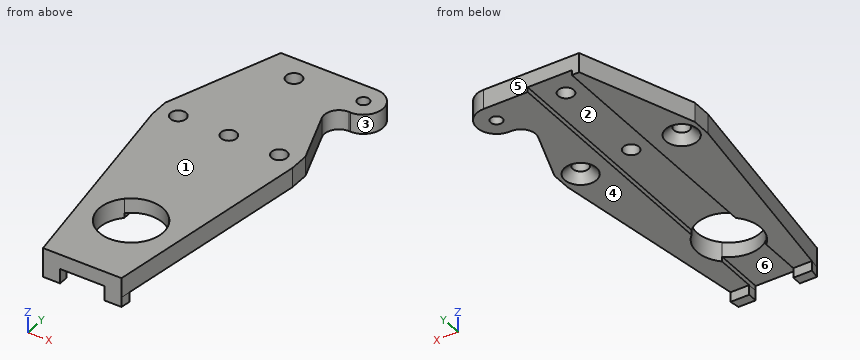
from build123d import *

# Parameters (mm, degrees)
MODEL_R           = 1.2
MODEL_R_2         = 1.6
EXTRUDE_4_DEPTH   = 4
EXTRUDE_4_2_DEPTH = 4
MODEL_7_R         = 1.6
EXTRUDE_5_DEPTH   = 3
EXTRUDE_6_DEPTH   = 6
CHAMFER_2_SIZE    = 1.65


with BuildPart() as part:
    # Model → Extrude 4 (new body)
    with BuildSketch(Plane.XY):
        with BuildLine():
            Line((36.699535099, 24.454545455), (37.040606061, 24.454545455))
            ThreePointArc((37.040606061, 24.454545455), (41.040606061, 28.454545455), (37.040606061, 32.454545455))
            Line((37.040606061, 32.454545455), (28.040606061, 32.454545455))
            Line((28.040606061, 32.454545455), (28.040606061, -17.855038786))
            ThreePointArc((28.040606061, -17.855038786), (30.040606061, -22.545454545), (28.040606061, -27.235870305))
            Line((28.040606061, -27.235870305), (28.040606061, -37.545454545))
            Line((28.040606061, -37.545454545), (31.540606061, -37.545454545))
            Line((31.540606061, -37.545454545), (37.840606061, 5.454545455))
            Line((37.840606061, 5.454545455), (37.840606061, 9.454545455))
            Line((37.840606061, 9.454545455), (33.877655721, 20.43621507))
            ThreePointArc((33.877655721, 20.43621507), (34.244439261, 23.178640702), (36.699535099, 24.454545455))
        make_face()
        with Locations((37.040606061, 28.454545455)):
            Circle(MODEL_R, mode=Mode.SUBTRACT)
        with Locations((33.840606061, 7.454545455)):
            Circle(MODEL_R_2, mode=Mode.SUBTRACT)
    extrude(amount=-EXTRUDE_4_DEPTH)



with BuildPart() as body_2:
    # Model → Extrude 4 2 (new body)
    with BuildSketch(Plane.XY):
        with BuildLine():
            Line((19.040606061, -17.855038786), (19.040606061, 32.454545455))
            Line((19.040606061, 32.454545455), (17.540606061, 32.454545455))
            Line((17.540606061, 32.454545455), (9.240606061, 9.454545455))
            Line((9.240606061, 9.454545455), (9.240606061, 5.454545455))
            Line((9.240606061, 5.454545455), (15.540606061, -37.545454545))
            Line((15.540606061, -37.545454545), (19.040606061, -37.545454545))
            Line((19.040606061, -37.545454545), (19.040606061, -27.235870305))
            ThreePointArc((19.040606061, -27.235870305), (17.040606061, -22.545454545), (19.040606061, -17.855038786))
        make_face()
        with Locations((13.240606061, 7.454545455)):
            Circle(MODEL_R_2, mode=Mode.SUBTRACT)
    extrude(amount=-EXTRUDE_4_2_DEPTH)


with BuildPart() as part_1:
    add(part.part)

    add(body_2.part)  # Extrude 5 merges body 2
    # Model_7 → Extrude 5 (add)
    # profile 1 of 2: a face of its own
    with BuildSketch(Plane.XY):
        with BuildLine():
            Line((28.040606061, -35.545454545), (28.040606061, -27.235870305))
            ThreePointArc((28.040606061, -27.235870305), (23.540606061, -29.045454545), (19.040606061, -27.235870305))
            Line((19.040606061, -27.235870305), (19.040606061, -35.545454545))
            Line((19.040606061, -35.545454545), (19.040606061, -37.545454545))
            Line((19.040606061, -37.545454545), (28.040606061, -37.545454545))
            Line((28.040606061, -37.545454545), (28.040606061, -35.545454545))
        make_face()
    # profile 2 of 2: a face of its own
    with BuildSketch(Plane.XY):
        with BuildLine():
            Line((28.040606061, -17.855038786), (28.040606061, 32.454545455))
            Line((28.040606061, 32.454545455), (19.040606061, 32.454545455))
            Line((19.040606061, 32.454545455), (19.040606061, -17.855038786))
            ThreePointArc((19.040606061, -17.855038786), (23.540606061, -16.045454545), (28.040606061, -17.855038786))
        make_face()
        with Locations((23.540606061, 7.454545455)):
            Circle(MODEL_7_R, mode=Mode.SUBTRACT)
        with Locations((23.540606061, 27.454545455)):
            Circle(MODEL_7_R, mode=Mode.SUBTRACT)
    extrude(amount=-EXTRUDE_5_DEPTH)

    # Model_8 → Extrude 6 (add)
    with BuildSketch(Plane.XY):
        Polygon((31.540606061, -37.545454545), (31.833629316, -35.545454545), (28.04060606, -35.545454545), (28.040606061, -37.545454545), align=None)
        Polygon((19.040606061, -37.545454545), (19.040606061, -35.545454545), (15.247582805, -35.545454545), (15.540606061, -37.545454545), align=None)
    extrude(amount=-EXTRUDE_6_DEPTH)

    # Chamfer 2
    chamfer_2_edges = [part_1.edges().sort_by_distance(p)[0] for p in [
        (32.240606061, 7.454545455, -4),
        (11.640606061, 7.454545455, -4),
    ]]
    chamfer(chamfer_2_edges, length=CHAMFER_2_SIZE)


solid = part_1.part
CAD build for the part. Positions are in the model's coordinates, mm. Face numbers are marked on the shaded views. A direction names the side the tool comes from. Round coordinates to 2 decimals unless told otherwise and drop trailing zeros. Loops run counter-clockwise (first coordinate to the right, second up) from the corner with the lowest first, then second, coordinate; pieces in that order, holes last. Notation, with made-up numbers: (-39, -15.5) - (17, -15.5) arc R7 cw to (17, -10.5) - close; hole circle Ø1 at (-20, -9.5). An arc over 180 degrees is marked (long way). Put each result on its own line as item: value.
1. 3-axis set-ups, long thin cutter, end or side, ignore diameter. For the marked faces 4, 5 and 6: which of +Z, -Z, +X, -X, +Y, -Y reach the whole face in a straight line?
Geometry check:
face 4: -Z, +X, -X, +Y
face 5: +Z, -Z, +X, -X, +Y
face 6: -Z, +Y, -Y
2. Slice it at A-A on y = -28. List the corners of the cut face in (x, z), and give its area (3 significant figures).
Geometry check:
outline: (14.14, -4) - (19.04, -4) - (19.04, -3) - (20.01, -3) - (20.01, 0) - (14.14, 0) - close; (27.08, -3) - (28.04, -3) - (28.04, -4) - (32.94, -4) - (32.94, 0) - (27.08, 0) - close
area: 45.0 mm²
3. Slice it at D-D on y = 3. List the corners of the cut face in (x, z).
Geometry check:
outline: (9.6, -4) - (19.04, -4) - (19.04, -3) - (28.04, -3) - (28.04, -4) - (37.48, -4) - (37.48, 0) - (9.6, 0) - close
4. Two-plate mould, pull along X, no slides. Class the marked faces 1, 2 and 3: released by +X, released by -X, zero draft, split by the parting line, or undercut.
Geometry check:
face 1: zero draft
face 2: undercut
face 3: released by +X
5. Pin check, flat tips, straight feed: P1, Ø10, axis at x = 20.5, y = 16, coming from the +Z side; P2, Ø14.5, axis at x = 37, y = -10, coming from the -Z side; P3, Ø0.8, axis at y = 7.5, z = -3.5, coming from the +X side; P4, Ø1.6, axis at x = 30.5, z = -5.5, coming from the +Y side. Stop position of each tip, or through.
Geometry check:
P1: z = 0
P2: z = -4
P3: x = 37.84
P4: y = -35.55
6. Wall check: line 1 (X direction, y = 27.5, z = -3.75); line 2 (Z direction, x = 25, y = 6); line 3 (Z direction, x = 33, y = -1.5). Give the ranges that are in metal, low to high.
Geometry check:
line 1: 15.75 to 19.04, 28.04 to 36.31, 37.77 to 40.93
line 2: -3 to 0
line 3: -4 to 0
7. Slice it at C-C on z = -0.8. List the corners of the cut face in (x, y), and give its area (3 significant figures).
Geometry check:
outline: (9.24, 5.45) - (15.54, -37.55) - (31.54, -37.55) - (37.84, 5.45) - (37.84, 9.45) - (33.88, 20.44) arc R3 cw to (36.7, 24.45) - (37.04, 24.45) arc R4 ccw to (37.04, 32.45) - (17.54, 32.45) - (9.24, 9.45) - close; hole circle Ø3.2 at (13.24, 7.45); hole circle Ø13 at (23.54, -22.55); hole circle Ø3.2 at (23.54, 7.45); hole circle Ø3.2 at (23.54, 27.45); hole circle Ø3.2 at (33.84, 7.45); hole circle Ø2.4 at (37.04, 28.45)
area: 1,450 mm²
8. Slice it at B-B on x = 29. List the corners of the cut face in (y, z).
Geometry check:
outline: (-37.55, -6) - (-35.55, -6) - (-35.55, -4) - (-26.07, -4) - (-26.07, 0) - (-37.55, 0) - close; (-19.02, -4) - (32.45, -4) - (32.45, 0) - (-19.02, 0) - close
